The model under review builds one solid part; all positions refer to its coordinate system, in mm. Face numbers are marked on the shaded views. Coordinates: 2 decimals unless noted, no trailing zeros. Write each loop counter-clockwise with the first axis right and the second up, starting at its lowest first coordinate (ties: lowest second). Pieces come first, ordered by that corner, then holes. Notation, with made-up numbers: M -29.75,-21.5 L -13.75,-21.5 A30 ccw -13.75,16.5 Z; hole C 73.25,3 d5. An arc over 180 degrees is marked long. Answer as a JSON object with one key per item and string values.
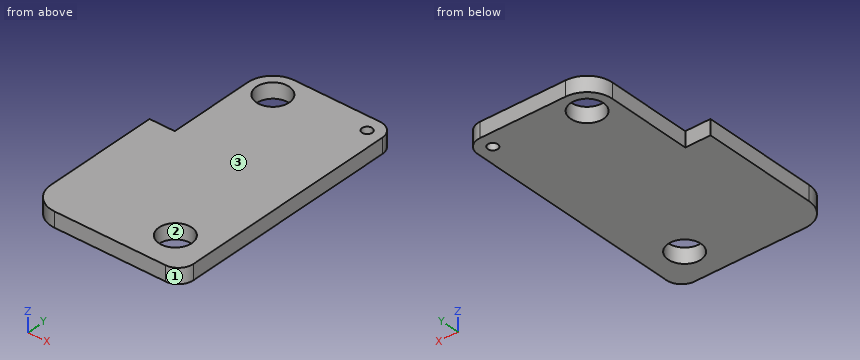
Autodesk Inventor part; units mm, degrees
ref_plane "YZ Plane" through (0, 0, 0) normal (1, 0, 0) x (0, 1, 0)
ref_plane "XZ Plane" through (0, 0, 0) normal (0, 1, 0) x (-1, 0, 0)
ref_plane "XY Plane" through (0, 0, 0) normal (0, 0, 1) x (1, 0, 0)
sketch "Sketch1" plane through (0, 0, 0) normal (0, 0, 1) x (1, 0, 0)
  line L0 (0, 0) -> (10, 0)
  line L1 (10, 0) -> (10, 10)
  line L2 (10, 10) -> (0, 10)
  line L3 (0, 10) -> (0, 0)
  line L4 (10, 10) -> (25, 10)
  line L5 (25, 10) -> (25, 4)
  line L6 (25, 4) -> (10, 4)
  line L7 (10, 4) -> (10, 10)
  line L8 (10, 0) -> (0, 0)
  line L9 (0, 0) -> (0, -40)
  line L10 (0, -40) -> (10, -40)
  line L11 (10, -40) -> (10, 0)
  line L12 (0, -40) -> (-5, -40)
  line L13 (-5, -40) -> (-5, -12)
  line L14 (-5, -12) -> (0, -12)
  line L15 (0, -12) -> (0, -40)
  line L16 (10, 4) -> (25, 4)
  line L17 (25, 4) -> (25, -40)
  line L18 (25, -40) -> (10, -40)
  line L19 (10, -40) -> (10, 4)
  dimension "d0" = 10
  dimension "d2" = 15
  dimension "d3" = 6
  dimension "d5" = 28
  dimension "d6" = 5
  dimension "d7" = 10
  dimension "d30" = 22
extrude "Extrusion1" add sketch "Sketch1" along normal blind 3
fillet "Fillet1" radius 5 1 edges at (0, 10, 1.5)
fillet "Fillet2" radius 5 1 edges at (-5, -40, 1.5)
fillet "Fillet3" [suppressed]
fillet "Fillet4" [suppressed]
sketch "Sketch2" plane through (0, 0, 3) normal (0, 0, 1) x (1, 0, 0)
  line L0 (25, 10) -> (5, 10)
  line L1 (25, -40) -> (25, 10)
  point P0 (0, 0)
  point P1 (22, 7)
  dimension "d33" = 3
  dimension "d34" = 3
hole "Hole1" at (22, 7, 3) direction (0, 0, -1) diameter 2 end through all
sketch "Sketch3" plane through (0, 0, 3) normal (0, 0, 1) x (1, 0, 0)
  line L0 (25, 10) -> (5, 10)
  line L1 (0, 5) -> (0, -12)
  line L2 (25, -40) -> (25, 10)
  line L3 (0, -40) -> (25, -40)
  point P0 (0, 0)
  point P1 (5, 5)
  point P2 (22, 10)
  point P3 (18, -33)
  dimension "d20" = 5
  dimension "d31" = 5
  dimension "d36" = 7
  dimension "d37" = 7
hole "Hole2" at (5, 5, 3) at (18, -33, 3) direction (0, 0, -1) diameter 6.5 end through all
fillet "Fillet6" radius 3 2 edges at (25, -40, 1.5) (25, 10, 1.5)
sketch "Sketch4" plane through (0, 0, 3) normal (0, 0, 1) x (1, 0, 0)
  point P0 (0, 0)
properties part number "Selection_Lever 1" material "Nylon 6/6"
(1) Add section A-A on y = -33. Give the boundary of the cut face in (x, z), and give its area (3 significant figures).
Results list:
{"outline": "M -5,0 L 14.75,0 L 14.75,3 L -5,3 Z; M 21.25,0 L 25,0 L 25,3 L 21.25,3 Z", "area": "70.5 mm²"}
(2) Add section C-C on x = 18. Give the boundary of the cut face in (y, z), and give its area (4 significant figures).
Results list:
{"outline": "M -40,0 L -36.25,0 L -36.25,3 L -40,3 Z; M -29.75,0 L 10,0 L 10,3 L -29.75,3 Z", "area": "130.5 mm²"}
(3) Add section D-D on y = -9. Give the boundary of the cut face in (x, z), and give its area (3 significant figures).
Results list:
{"outline": "M 0,0 L 25,0 L 25,3 L 0,3 Z", "area": "75.0 mm²"}
(4) Draft analysis for pull direction Y (two halves, no side actions). For the marked faces 1, 2 and 3, state which applies: released by +Y, released by -Y, zero draft, split by the parting line, or undercut.
Results list:
{"face 1": "released by -Y", "face 2": "undercut", "face 3": "zero draft"}
(5) Add section B-B on z = 2.4. Give the boundary of the cut face in (x, y), and give its area (3 significant figures).
Results list:
{"outline": "M -5,-35 A5 ccw 0,-40 L 22,-40 A3 ccw 25,-37 L 25,7 A3 ccw 22,10 L 5,10 A5 ccw 0,5 L 0,-12 L -5,-12 Z; hole C 5,5 d6.5; hole C 18,-33 d6.5; hole C 22,7 d2", "area": "1,310 mm²"}
(6) Wall thickness on line 1 along Y through (x, z) = (22, 1.6); line 2 along Y through (x, z) = (18, 1.4); line 3 along X through (y, z) = (-33, 1.45): over which ranges is each line inside the solid? List them lowest first. Write a range as from..to.
Results list:
{"line 1": "-40..6, 8..10", "line 2": "-40..-36.25, -29.75..10", "line 3": "-5..14.75, 21.25..25"}
(7) For pin 1 Ø1.5 at (y, z) = (-7.5, 1.5) entering from -X; pin 2 Ø1.5 at (x, z) = (-1.5, 2) entering from +Y, all flat-tipped, find the tip position at first contact; note any pin that passes through.
Results list:
{"pin 1": "x = 0", "pin 2": "y = -12"}
